from build123d import *

# Parameters (mm, degrees)
SKETCH1_W            = 52
SKETCH1_H            = 52
SKETCH1_R            = 12
BOSS_EXTRUDE1_DEPTH  = 3
SKETCH2_W            = 52
SKETCH2_H            = 41
BOSS_EXTRUDE2_DEPTH  = 3
M3_CLEARANCE_HOLE1_D = 3.4
M4_CLEARANCE_HOLE1_D = 4.5
BOSS_EXTRUDE3_DEPTH  = 3
BOSS_EXTRUDE4_DEPTH  = 3
FILLET1_R            = 2


with BuildPart() as part:
    # Sketch1 → Boss-Extrude1 (new body)
    with BuildSketch(Plane(origin=(0, 0, 0), x_dir=(1, 0, 0), z_dir=(0, 1, 0))):
        with Locations((-3, 0)):
            Rectangle(SKETCH1_W, SKETCH1_H)
        with Locations(Location((0, 0, 0), (0, 0, 270))):
            Circle(SKETCH1_R, mode=Mode.SUBTRACT)
    extrude(amount=BOSS_EXTRUDE1_DEPTH)

    # Sketch2 → Boss-Extrude2 (add)
    with BuildSketch(Plane.ZY.offset(29)):
        with Locations((0, -20.5)):
            Rectangle(SKETCH2_W, SKETCH2_H)
    extrude(amount=-BOSS_EXTRUDE2_DEPTH)

    # M3 Clearance Hole1 (through all)
    with Locations(Plane(origin=(0, 3, 0), x_dir=(1, 0, 0), z_dir=(0, 1, 0))):
        with Locations((15.494, -15.494), (-15.494, -15.494), (-15.494, 15.494), (15.494, 15.494)):
            Hole(M3_CLEARANCE_HOLE1_D / 2)

    # M4 Clearance Hole1 (through all)
    with Locations(Plane(origin=(-26, 0, 0), x_dir=(0, 0, -1), z_dir=(1, 0, 0))):
        with Locations((-10, -9), (10, -9), (10, -31), (-10, -31), (0, -9), (0, -31)):
            Hole(M4_CLEARANCE_HOLE1_D / 2)

    # Sketch7 → Boss-Extrude3 (add)
    with BuildSketch(Plane(origin=(0, 0, -26), x_dir=(-1, 0, 0), z_dir=(0, 0, -1))):
        Polygon((26, -41), (-23, 0), (26, 0), align=None)
    extrude(amount=-BOSS_EXTRUDE3_DEPTH)

    # Sketch8 → Boss-Extrude4 (add)
    with BuildSketch(Plane.XY.offset(26)):
        Polygon((23, 0), (-26, -41), (-26, 0), align=None)
    extrude(amount=-BOSS_EXTRUDE4_DEPTH)

    # Fillet1
    fillet1_edges = [part.edges().sort_by_distance(p)[0] for p in [
        (-1.5, -20.5, 26),
        (-1.5, -20.5, -26),
    ]]
    fillet(fillet1_edges, radius=FILLET1_R)


solid = part.part
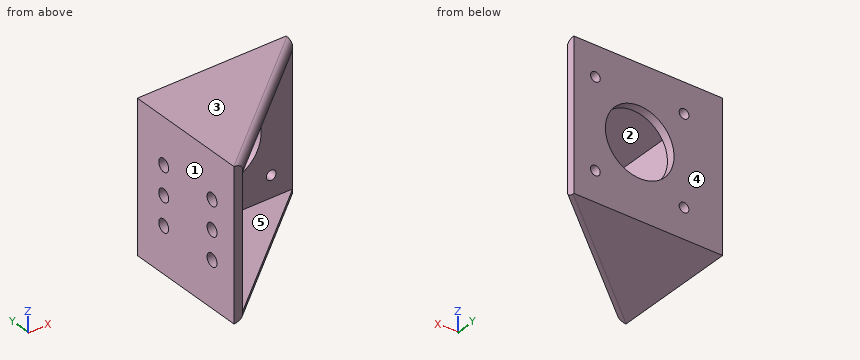
Input: part model. Units: mm. Frame: model coordinates. Face numbers are marked on the shaded views. A direction names the side the tool comes from. Round coordinates to 2 decimals unless told otherwise and drop trailing zeros. Loops run counter-clockwise (first coordinate to the right, second up) from the corner with the lowest first, then second, coordinate; pieces in that order, holes last. Notation, with made-up numbers: M 14,14.25 L 56,14.25 A28 cw 56,51.25 Z; hole C 87.5,69 d9. An arc over 180 degrees is marked long. Answer as CSV lines item,"result". Start each with the question number.
(1) Section B-B, the plane z = 22. Output: boundary loops of the cut face in (x, y), plus the area to 3 significant figures.
(2) Section D-D, the plane z = -10. Output: boundary loops of the cut face in (x, y), plus the area to 3 significant figures.
(3) Section C-C, the plane y = -31. State how many separate pieces and enclosed holes the cut face has, plus the area to 3 significant figures.
(4) Line query: line 1 (Y direction, x = -27, z = -10); line 2 (Z direction, x = 0.5, y = 1.5); line 3 (Z direction, x = -12, y = -16). Output: solid intervals per line, ascending. Write a range as [from, to].
(5) Draft query along Z for the marked faces 1, 2 and 3. Return one class per face: released by +Z, released by -Z, zero draft, split by the parting line, or undercut.
(6) First-contact query: pin 1 (6 mm diameter, centred on y = -31, z = -10, fed in from +X); pin 2 (23 mm diameter, centred on x = 1.5, z = 4, fed in from -Y). Flat tips, straight axial feed; report the tip coordinate or a pass-through.
(7) Section A-A, the plane z = 0. Output: boundary loops of the cut face in (x, y), plus the area to 3 significant figures.
(8) Reachability of the marked faces 4 and 5 from +Z, -Z, +X, -X, +Y, -Y: full face, straight path, thin tool, end or side. Return the list, or none.
Values found:
1,outline,"M -29,-41 L -26,-41 L -26,0 L 23,0 L 23,3 L -29,3 Z"
1,area,"279 mm²"
2,outline,"M -29,-41 L -26,-41 L -26,-33.25 L -29,-33.25 Z; M -29,-28.75 L -26,-28.75 L -26,-11.25 L -29,-11.25 Z; M -29,-6.75 L -26,-6.75 L -26,0 L -6.63,0 L -6.63,3 L -29,3 Z; M 6.63,0 L 23,0 L 23,3 L 6.63,3 Z"
2,area,"212 mm²"
3,separate pieces,"4"
3,enclosed holes,"0"
3,area,"185 mm²"
4,line 1,"y = [-41, -33.25], [-28.75, -11.25], [-6.75, 3]"
4,line 2,"z = [-26, -11.99], [11.99, 26]"
4,line 3,"z = [-26, -23], [23, 26]"
5,face 1,"zero draft"
5,face 2,"undercut"
5,face 3,"released by +Z"
6,pin 1,"stops at x = -26"
6,pin 2,"stops at y = 0"
7,outline,"M -29,-41 L -26,-41 L -26,-33.25 L -29,-33.25 Z; M -29,-28.75 L -26,-28.75 L -26,-11.25 L -29,-11.25 Z; M -29,-6.75 L -26,-6.75 L -26,0 L -12,0 L -12,3 L -29,3 Z; M 12,0 L 23,0 L 23,3 L 12,3 Z"
7,area,"180 mm²"
8,face 4,"+Z, -Z, +X, -X, +Y"
8,face 5,"+X, -Y"
